```python
from build123d import *

# Parameters (mm, degrees)
SKETCH7_W           = 18
SKETCH7_H           = 46
SKETCH8_R           = 18
SKETCH8_R_2         = 11
BOSS_EXTRUDE1_DEPTH = 17.5


with BuildPart() as part:
    # Sketch1 → Revolve1 (revolve)
    with BuildSketch(Plane.XY, mode=Mode.PRIVATE) as revolve1_sk:
        with BuildLine():
            Line((37, 0), (46, 0))
            Line((46, 0), (46, 5))
            Line((46, 5), (42, 5))
            Line((42, 5), (42, 7))
            Line((42, 7), (46, 7))
            Line((46, 7), (46, 45))
            Line((46, 45), (42, 45))
            Line((42, 45), (42, 48))
            Line((42, 48), (46, 48))
            Line((46, 48), (46, 50))
            Line((46, 50), (42, 50))
            Line((42, 50), (42, 53))
            Line((42, 53), (46, 53))
            Line((46, 53), (46, 55))
            Line((46, 55), (42, 55))
            Line((42, 55), (42, 58))
            Line((42, 58), (46, 58))
            Line((46, 58), (46, 60))
            Line((46, 60), (42, 60))
            Line((42, 60), (42, 63))
            Line((42, 63), (46, 63))
            Line((46, 63), (46, 65))
            ThreePointArc((46, 65), (23.180726365, 69.327783179), (0, 70.777914783))
            Line((0, 70.777914783), (0, 62))
            Line((0, 62), (37, 62))
            Line((37, 62), (37, 0))
        make_face()
    revolve(revolve1_sk.sketch.rotate(Axis((0, 70.777914783, 0), (0, -1, 0)), 180), axis=Axis((0, 70.777914783, 0), (0, -1, 0)))

    # Sketch7 → Ø12.0mm Dowel Hole3 (revolve, cut)
    with BuildSketch(Plane(origin=(0, 25.5, 0), x_dir=(0, 1, 0), z_dir=(1, 0, 0))):
        with Locations((9, 23)):
            Rectangle(SKETCH7_W, SKETCH7_H)
    f_12_0mm_dowel_hole3 = revolve(axis=Axis((0, 25.5, -6.35), (0, 0, 1)), mode=Mode.SUBTRACT)

    # Sketch8 → Boss-Extrude1 (add)
    with BuildSketch(Plane.XY.offset(25)):
        with Locations(Location((0, 25.5, 0), (0, 0, 180))):
            Circle(SKETCH8_R)
        with Locations((0, 25.5)):
            Circle(SKETCH8_R_2, mode=Mode.SUBTRACT)
    boss_extrude1 = extrude(amount=BOSS_EXTRUDE1_DEPTH)

    # Mirror1: Ø12.0mm Dowel Hole3, Boss-Extrude1 across plane
    add(f_12_0mm_dowel_hole3.mirror(Plane.XY), mode=Mode.SUBTRACT)
    add(boss_extrude1.mirror(Plane.XY))


solid = part.part
```
Read the model definition and answer for the solid it produces. Units are mm, in the model's axes. A direction names the side the tool comes from. Give positions to 0.01 mm unless a question says otherwise; leave off trailing zeros. Write each loop counter-clockwise with the first axis right and the second up, starting at its lowest first coordinate (ties: lowest second). Pieces come first, ordered by that corner, then holes. Notation, with made-up numbers: (46.5, 75.25) - (54.5, 75.25) arc R14 ccw to (54.5, 93.25) - close; hole circle Ø9 at (-35, 25). An arc over 180 degrees is marked (long way). Write item = value, one per line. Start each with the question number.
Item 1: Each of these flat-tipped pins is pushed along its axis until it touches: P1, Ø18, axis at x = -3.5, y = 17, coming from the +Z side; P2, Ø10, axis at y = 51, z = 25.5, coming from the -X side; P3, Ø5, axis at y = 46, z = 9.5, coming from the -X side. Where does it stop, or does it pass through?
Item 2: The mould has two halves that part along X. Classify faces 4 (the cylindrical face through (-0.343, 7.503, 43.886)), 5 (the cylindrical face through (-40.06, 61.52, -12.62)), 6 (the flat face through (-20.2, 50, 37.3)): +X half, -X half, draft (parallel to the pull), parting line (faces both ways), or undercut.
Item 3: A tool of negligible diameter and unlimited length cuts with its end or side. For faces 1 (the cylindrical face through (0.343, 43.497, 43.886)), 2 (the flat face through (8.3, 33.2, -42.5)), 3 (the cylindrical face through (-40.06, 46.52, -12.62)), from which of +Z, -Z, +X, -X, +Y, -Y can it reach the whole face along a straight path? Write none if from no direction.
Item 4: Find section C-C (x = 4). State how many separate pieces and enclosed holes the cut face has, then the cut area to 3 significant figures.
Item 5: Find section B-B (y = 10). Give the vertices of the cut face in (x, z).
Item 6: Find section A-A (y = 25.5). Give the vertices of the cut face in (x, z), then the cut area to 3 significant figures.
Item 7: Find the intervals of material crossed by probe 1 along Z at (x, y) = (0, 42.5); probe 2 along Y at (x, z) = (-5, -31); probe 3 along Y at (x, z) = (1, -33), in increasing order. Write a range as [from, to].
Response:
q1.P1 = 45.79
q1.P2 = -41.13
q1.P3 = -45.43
q2.face_4 = undercut
q2.face_5 = parting line
q2.face_6 = draft
q3.face_1 = +Z
q3.face_2 = -Z
q3.face_3 = none
q4.separate_pieces = 3
q4.enclosed_holes = 0
q4.area = 1,510 mm²
q5.outline = (-9.15, -45.08) - (-9.15, -42.5) - (9.15, -42.5) - (9.15, -45.08) arc R46 ccw to (9.15, 45.08) - (9.15, 42.5) - (-9.15, 42.5) - (-9.15, 45.08) arc R46 ccw to start; hole (-9.15, -35.85) - (-9.15, -25) - (9.15, -25) - (9.15, -35.85) arc R37 ccw to (9.15, 35.85) - (9.15, 25) - (-9.15, 25) - (-9.15, 35.85) arc R37 ccw to start
q6.outline = (-18, -42.5) - (-11, -42.5) - (-11, -25) - (-18, -25) - (-18, -32.33) arc R37 cw to (-18, 32.33) - (-18, 25) - (-11, 25) - (-11, 42.5) - (-18, 42.5) - (-18, 42.33) arc R46 ccw to (-18, -42.33) - close; (11, -42.5) - (18, -42.5) - (18, -42.33) arc R46 ccw to (18, 42.33) - (18, 42.5) - (11, 42.5) - (11, 25) - (18, 25) - (18, 32.33) arc R37 cw to (18, -32.33) - (18, -25) - (11, -25) - close
q6.area = 2,170 mm²
q7.probe_1 = [-42.5, -25], [25, 42.5]
q7.probe_2 = [8.21, 15.7], [35.3, 42.79], [62, 68.11]
q7.probe_3 = [7.53, 14.55], [36.45, 43.47], [62, 67.82]
